```python
from build123d import *

# Parameters (mm, degrees)
F0_W          = 11
F0_H          = 15
F1_DEPTH      = 1.3
F0_W_2        = 3
F2_DEPTH      = 7
F3_SIZE       = 2
F5_DEPTH      = 2.5
F5_DEPTH_BACK = 16.5


with BuildPart() as f1:
    # F0 (on Top) → F1 (new body)
    with BuildSketch(Plane.XY):
        Polygon((22.3, -115.8), (22.3, -100), (-28, -100), (-28, -133.8), (22.3, -133.8), (22.3, -130.8), (11.3, -130.8), (11.3, -115.8), align=None)
        with Locations((16.8, -123.3)):
            Rectangle(F0_W, F0_H)
    extrude(amount=-F1_DEPTH)

    # F0 (on Top) → F2 (join)
    with BuildSketch(Plane.XY):
        with Locations((23.8, -123.3)):
            Rectangle(F0_W_2, F0_H)
        with Locations((16.8, -123.3)):
            Rectangle(F0_W, F0_H)
    extrude(amount=F2_DEPTH)

    # F3
    f3_edges = [f1.edges().sort_by_distance(p)[0] for p in [
        (22.3, -133.8, -0.65),
        (-28, -133.8, -0.65),
        (22.3, -100, -0.65),
        (-28, -100, -0.65),
    ]]
    chamfer(f3_edges, length=F3_SIZE)

    # F4 (on face) → F5 (join, two sides)
    with BuildSketch(Plane(origin=(0, 0, -1.3), x_dir=(1, 0, 0), z_dir=(0, 0, -1))) as f5_sk:
        Polygon((-25.751472, 133.2), (-27.4, 131.551472), (-27.4, 102.5), (-21, 102.5), (-21, 100.6), (20.051472, 100.6), (21.7, 102.248528), (21.7, 131.551472), (20.051472, 133.2), (3.3, 133.2), (3.3, 128.2), (-4.7, 128.2), (-4.7, 133.2), align=None)
    extrude(amount=F5_DEPTH)
    extrude(f5_sk.sketch, amount=-F5_DEPTH_BACK)


with BuildPart() as f1_1:
    # F6: moved
    add(f1.part.moved(Location((0, 0, 4))))


solid = f1_1.part
```
The model under review builds one solid part; all positions refer to its coordinate system, in mm. A direction names the side the tool comes from. Give positions to 0.01 mm unless a question says otherwise; leave off trailing zeros. Write each loop counter-clockwise with the first axis right and the second up, starting at its lowest first coordinate (ties: lowest second). Pieces come first, ordered by that corner, then holes. Notation, with made-up numbers: (-15, -25) -> (40, -25) arc R33 ccw to (40, 8) -> close; hole circle Ø4 at (-9.5, 69.5). An arc over 180 degrees is marked (long way). Answer in a Markdown table with one row per item.
1) For L1, parallel to X at y = -129.5, z = 14.5; L2, parallel to Y at x = 8.5, z = 12.25; L3, parallel to X at y = -111, z = 15.75, list the stretches that pass through material, from the lowest coordinate up. Write a range as [from, to].
Worked answers:
| item | result |
|---|---|
| L1 | [-27.4, -4.7], [3.3, 21.7] |
| L2 | [-133.2, -100.6] |
| L3 | [-27.4, 21.7] |
2) Tool access review of faces 1 (the flat face through (-24, -102.5, 11)), 2 (the flat face through (20.89, -132.36, 1.47)), 3 (the flat face through (20.86, -101.41, 1.47)), 4 (the flat face through (-24, -102.5, 1)), 5 (the flat face through (-4.7, -131, 11)): name each direction out of +Z, -Z, +X, -X, +Y, -Y from which nothing blocks a thin tool from reaching the whole face with its end or side.
Worked answers:
| item | result |
|---|---|
| face 1 | +Z, -X, +Y |
| face 2 | -Z, +X, -Y |
| face 3 | -Z, +X, +Y |
| face 4 | -Z, -X, +Y |
| face 5 | +Z, -Y |
3) Mouldability with a two-part tool opening along X and no side actions: class faces 6 (the flat face through (24, -123, 4)), 7 (the flat face through (3.3, -131, 11)), 8 (the flat face through (20.89, -132.36, 11.49)) as +X half, -X half, draft (parallel to the pull), parting line (faces both ways), or undercut.
Worked answers:
| item | result |
|---|---|
| face 6 | draft |
| face 7 | undercut |
| face 8 | +X half |
4) Clearance check with flat-ended pins moving along their axes: P1, Ø4.5, axis at y = -114, z = 12.5, coming from the -X side; P2, Ø1.5, axis at y = -108, z = 17, coming from the +X side; P3, Ø5, axis at x = -25.5, z = 12, coming from the +Y side. State where each tip first meets the part, or that it passes through.
Worked answers:
| item | result |
|---|---|
| P1 | x = -27.4 |
| P2 | x = 21.7 |
| P3 | y = -102.5 |
5) Add section D-D on y = -121.5. State the section outline as (x, z) points, plus the area to 3 significant figures.
Worked answers:
| item | result |
|---|---|
| outline | (-28, 2.7) -> (-27.4, 2.7) -> (-27.4, 0.2) -> (21.7, 0.2) -> (21.7, 2.7) -> (22.3, 2.7) -> (22.3, 4) -> (25.3, 4) -> (25.3, 11) -> (21.7, 11) -> (21.7, 19.2) -> (-27.4, 19.2) -> (-27.4, 4) -> (-28, 4) -> close |
| area | 960 mm² |
6) Add section A-A on x = -12. State the section outline as (y, z) points.
Worked answers:
| item | result |
|---|---|
| outline | (-133.8, 2.7) -> (-133.2, 2.7) -> (-133.2, 0.2) -> (-100.6, 0.2) -> (-100.6, 2.7) -> (-100, 2.7) -> (-100, 4) -> (-100.6, 4) -> (-100.6, 19.2) -> (-133.2, 19.2) -> (-133.2, 4) -> (-133.8, 4) -> close |
7) Add section B-B on y = -114.5. State the section outline as (x, z) points.
Worked answers:
| item | result |
|---|---|
| outline | (-28, 2.7) -> (-27.4, 2.7) -> (-27.4, 0.2) -> (21.7, 0.2) -> (21.7, 2.7) -> (22.3, 2.7) -> (22.3, 4) -> (21.7, 4) -> (21.7, 19.2) -> (-27.4, 19.2) -> (-27.4, 4) -> (-28, 4) -> close |
8) Add section C-C on z = 10. State the section outline as (x, y) points, plus the area to 3 significant figures.
Worked answers:
| item | result |
|---|---|
| outline | (-27.4, -131.55) -> (-25.75, -133.2) -> (-4.7, -133.2) -> (-4.7, -128.2) -> (3.3, -128.2) -> (3.3, -133.2) -> (20.05, -133.2) -> (21.7, -131.55) -> (21.7, -130.8) -> (25.3, -130.8) -> (25.3, -115.8) -> (21.7, -115.8) -> (21.7, -102.25) -> (20.05, -100.6) -> (-21, -100.6) -> (-21, -102.5) -> (-27.4, -102.5) -> close |
| area | 1,600 mm² |
